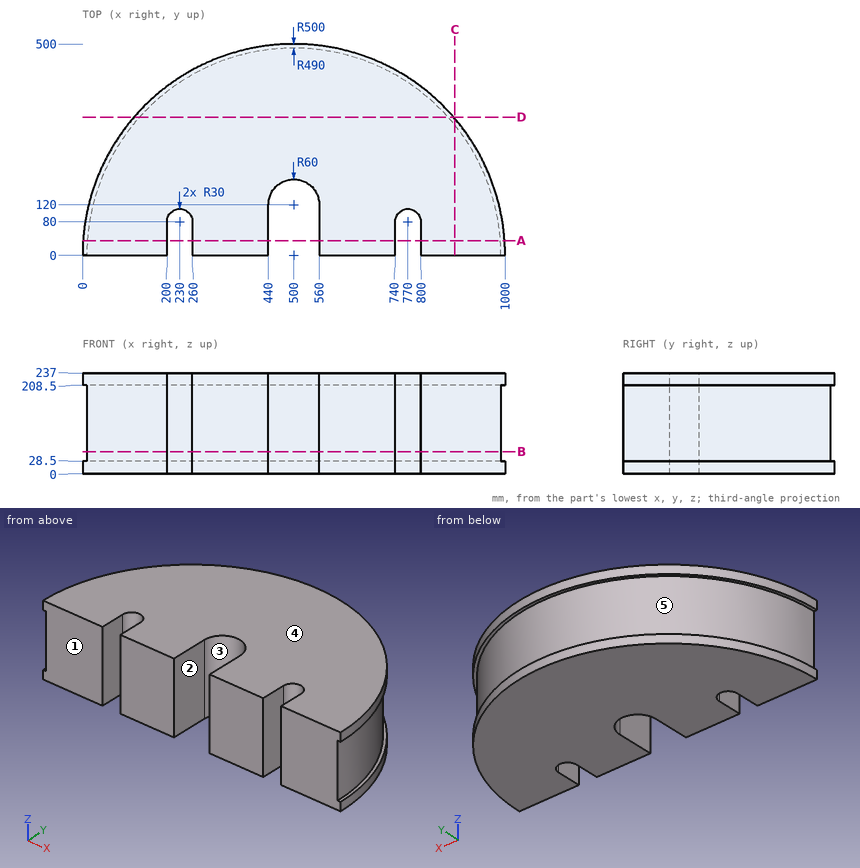
Input: dimensioned drawing with shaded views. Units: mm. Origin: part minimum x, y, z. A direction names the side the tool comes from. Give positions to 0.01 mm unless a question says otherwise; leave off trailing zeros. Write each loop counter-clockwise with the first axis right and the second up, starting at its lowest first coordinate (ties: lowest second). Pieces come first, ordered by that corner, then holes.
Q1. Section D-D, the plane y = 327. Output: boundary loops of the cut face in (x, z).
Q2. Section B-B, the plane z = 51.5. Output: boundary loops of the cut face in (x, y).
Q3. Material intervals for probe 1 along X at (y, z) = (98.5, 158); probe 2 along Z at (x, y) = (187.5, 377.5); probe 3 along X at (y, z) = (111.5, 206.5), sorted ascending.
Q4. Section A-A, the plane y = 35. Output: boundary loops of the cut face in (x, z).
Q5. Section C-C, the plane x = 881. Output: boundary loops of the cut face in (y, z), plus the area to 3 significant figures.
Q6. First-contact query: P1, Ø6, axis at x = 251, z = 158, coming from the -Y side; P2, Ø12, axis at x = 210.5, z = 136, coming from the -Y side; P3, Ø8, axis at x = 208, z = 31, coming from the -Y side. Flat tips, straight axial feed; report the tip coordinate or a pass-through.
Q7. Set-up query: the marked faces 1 and 2. Return all of +Z, -Z, +X, -X, +Y, -Y with unobstructed straight access to the full face (end or side cutting, diameter ignored); none if empty.
Q8. Pull-direction query (X, two-part tool) for the marked faces 3, 4 and 5; classes: pulls with the +X half, pulls with the -X half, needs draft (parallel to the pull), parting line crosses it, or undercut.
Filled in:
1. outline: (121.75, 0) - (878.25, 0) - (878.25, 28.5) - (864.93, 28.5) - (864.93, 208.5) - (878.25, 208.5) - (878.25, 237) - (121.75, 237) - (121.75, 208.5) - (135.07, 208.5) - (135.07, 28.5) - (121.75, 28.5) - close
2. outline: (10, 0) - (200, 0) - (200, 80) arc R30 cw to (260, 80) - (260, 0) - (440, 0) - (440, 120) arc R60 cw to (560, 120) - (560, 0) - (740, 0) - (740, 80) arc R30 cw to (800, 80) - (800, 0) - (990, 0) arc R490 ccw to start
3. probe 1: x = 20 to 206.38, 253.62 to 440, 560 to 746.38, 793.62 to 980
3. probe 2: z = 0 to 28.5, 208.5 to 237
3. probe 3: x = 22.85 to 440, 560 to 977.15
4. outline: (1.23, 0) - (200, 0) - (200, 237) - (1.23, 237) - (1.23, 208.5) - (11.25, 208.5) - (11.25, 28.5) - (1.23, 28.5) - close; (260, 0) - (440, 0) - (440, 237) - (260, 237) - close; (560, 0) - (740, 0) - (740, 237) - (560, 237) - close; (800, 0) - (998.77, 0) - (998.77, 28.5) - (988.75, 28.5) - (988.75, 208.5) - (998.77, 208.5) - (998.77, 237) - (800, 237) - close
5. outline: (0, 0) - (323.79, 0) - (323.79, 28.5) - (308.12, 28.5) - (308.12, 208.5) - (323.79, 208.5) - (323.79, 237) - (0, 237) - close
5. area: 73,900 mm2
6. P1: stops at y = 98
6. P2: stops at y = 95.8
6. P3: stops at y = 94.97
7. face 1: +Z, -Z, +X, -X, -Y
7. face 2: +Z, -Z, -Y
8. face 3: undercut
8. face 4: needs draft
8. face 5: parting line crosses it
